Work out the finished part from the listing and answer in its coordinate system (mm). Give positions to 0.01 mm unless a question says otherwise; leave off trailing zeros. Order: outer loops, then holes, each group sorted by start corner. A loop starts at its lowest first (then second) coordinate and runs counter-clockwise, first axis right, second up. Notation, with made-up numbers: (70.5, -37.5) - (94.5, -37.5) arc R9 ccw to (94.5, -28.5) - close; hole circle Ø3 at (-10, 19.25). An arc over 180 degrees is marked (long way). Write each question's results on one line, items separated by ' | '.
Autodesk Inventor part; units mm, degrees
ref_plane "YZ Plane" through (0, 0, 0) normal (1, 0, 0) x (0, 1, 0)
ref_plane "XZ Plane" through (0, 0, 0) normal (0, 1, 0) x (-1, 0, 0)
ref_plane "XY Plane" through (0, 0, 0) normal (0, 0, 1) x (1, 0, 0)
sketch "Sketch1" plane through (0, 0, 0) normal (0, 1, 0) x (-1, 0, 0)
  circle A0 centre (0, 0) radius 127
  dimension "d0" = 254
extrude "Extrusion1" add sketch "Sketch1" along normal blind 6.35
sketch "Sketch2" plane through (0, 6.35, 0) normal (0, 1, 0) x (1, 0, 0)
  point P0 (0, 0)
  point P1 (0, 0)
hole "Hole1" at (0, 6.35, 0) direction (0, -1, 0) diameter 6.0452 end through all
sketch "Sketch3" plane through (0, 6.35, 0) normal (0, 1, 0) x (1, 0, 0)
  circle A0 centre (0, 0) radius 3.0226
  circle A1 centre (0, 0) radius 101.6
  point P0 (-101.6, 0)
  point P1 (0, -101.6)
  point P2 (0, 101.6)
  point P3 (101.6, 0)
  dimension "d10" = 203.2
hole "Hole2" at (-101.6, 6.35, 0) at (0, 6.35, 101.6) at (0, 6.35, -101.6) at (101.6, 6.35, 0) direction (0, -1, 0) diameter 9.8044 end through all
properties part number "Keep Out RSX Deck"
1. Straight lines are drawn through the part: line 1 (Z direction, x = 0, y = 2.5); line 2 (X direction, y = 5, z = -106); line 3 (Z direction, x = 101.5, y = 6.25). For each, find the intervals that lie inside material, in ascending order. Write a range as [from, to].
Answer list:
line 1: [-127, -106.5], [-96.7, -3.02], [3.02, 96.7], [106.5, 127] | line 2: [-69.95, -2.16], [2.16, 69.95] | line 3: [-76.33, -4.9], [4.9, 76.33]
2. Determine the mould class of faces 1 (the face through (-26, 6.35, 2)), 2 (the face through (1.878, 3.131, -97.072)), 3 (the face through (27.53, 3.13, 123.98)) for opening direction X: +X half, -X half, draft (parallel to the pull), parting line (faces both ways), or undercut.
Answer list:
face 1: draft | face 2: undercut | face 3: parting line
3. Given P1, Ø1, axis at y = 2, z = 84, coming from the +X side; P2, Ø1, axis at x = -33.5, y = 4.5, coming from the -Z side, each flat-ended and moving along its own axis, determine where each tip first touches the part or whether it passes through.
Answer list:
P1: x = 95.69 | P2: z = -122.64
4. A cutting plane is placed at D-D, the plane y = 2.5. Write down the section's boundary in (x, z).
Answer list:
outline: circle Ø254 at (0, 0); hole circle Ø9.8 at (-101.6, 0); hole circle Ø9.8 at (0, -101.6); hole circle Ø9.8 at (0, 101.6); hole circle Ø6.05 at (0, 0); hole circle Ø9.8 at (101.6, 0)
5. A cutting plane is placed at C-C, the plane z = -101.6. Write down the section's boundary in (x, y).
Answer list:
outline: (-76.2, 0) - (-4.9, 0) - (-4.9, 6.35) - (-76.2, 6.35) - close; (4.9, 0) - (76.2, 0) - (76.2, 6.35) - (4.9, 6.35) - close
6. A cutting plane is placed at A-A, the plane x = 101.6. Write down the section's boundary in (y, z).
Answer list:
outline: (0, -76.2) - (6.35, -76.2) - (6.35, -4.9) - (0, -4.9) - close; (0, 4.9) - (6.35, 4.9) - (6.35, 76.2) - (0, 76.2) - close
7. A cutting plane is placed at B-B, the plane x = 0. Write down the section's boundary in (y, z), then the cut area to 3 significant figures.
Answer list:
outline: (0, -127) - (6.35, -127) - (6.35, -106.5) - (0, -106.5) - close; (0, -96.7) - (6.35, -96.7) - (6.35, -3.02) - (0, -3.02) - close; (0, 3.02) - (6.35, 3.02) - (6.35, 96.7) - (0, 96.7) - close; (0, 106.5) - (6.35, 106.5) - (6.35, 127) - (0, 127) - close | area: 1,450 mm^2
